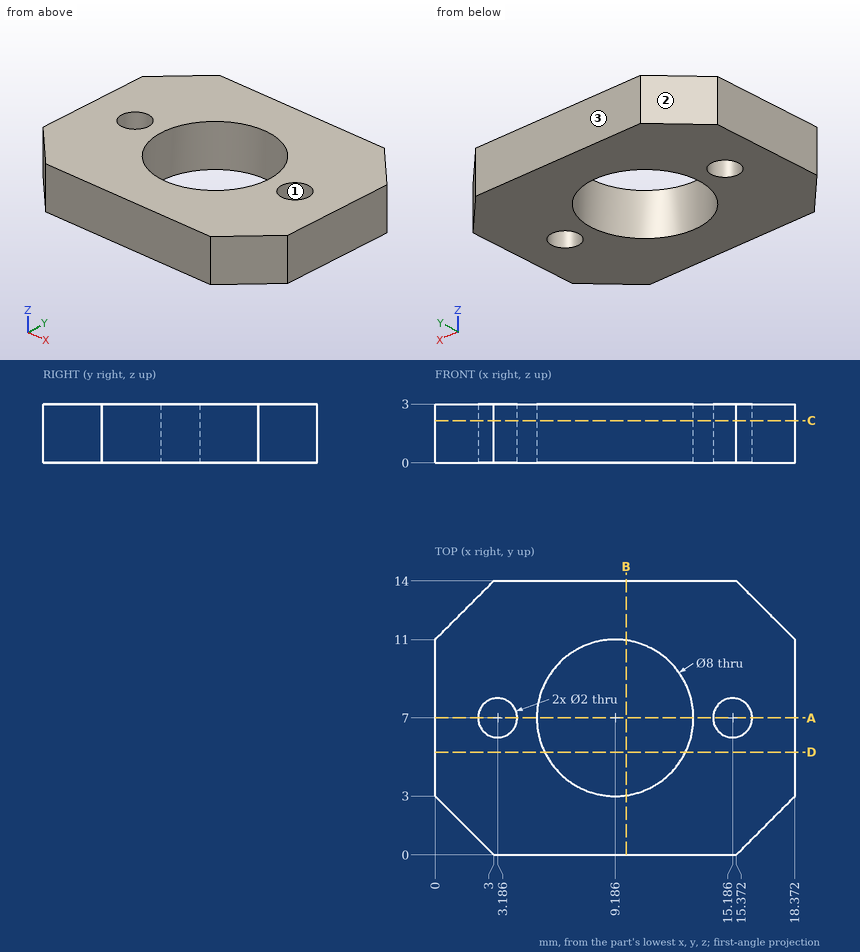
For this review, use the dimensioned drawing (mm, ordinates from the lowest corner) and the shaded views. Give positions to 0.01 mm unless a question says otherwise; leave off trailing zeros. Order: outer loops, then holes, each group sorted by start corner. A loop starts at its lowest first (then second) coordinate and runs counter-clockwise, first axis right, second up. Notation, with made-up numbers: (72.5, 82) - (86.5, 82) arc R19 ccw to (86.5, 110) - close; hole circle Ø10 at (35.25, 17.5). An arc over 180 degrees is marked (long way). Write item = value, one per line. Start each with the question number.
Q1. We need section D-D on y = 5.25. State the section outline as (x, z) points, plus the area to 3 significant figures.
Q2. Clearance check with flat-ended pins moving along their axes: pin 1 Ø2.5 at (x, y) = (15.19, 7) entering from +Z; pin 2 Ø1.6 at (x, y) = (3.19, 7) entering from -Z. State where each tip first meets the part, or that it passes through.
Q3. We need section A-A on y = 7. State the section outline as (x, z) points.
Q4. Mouldability with a two-part tool opening along X and no side actions: class the marked faces 1, 2 and 3 as released by +X, released by -X, zero draft, split by the parting line, or undercut.
Q5. We need section B-B on x = 9.75. State the section outline as (y, z) points, plus the area to 3 significant figures.
Q6. We need section C-C on z = 2.15. State the section outline as (x, y) points.
Q7. To check wall thickness, follow L1, parallel to X at y = 7.25, z = 1.6; L2, parallel to X at y = 9.75, z = 2.3; L3, parallel to Y at x = 8, z = 1.3. State the ranges of each line that lie inside material, in increasing order. Write a range as from..to.
Working result:
q1.outline = (0, 0) - (5.59, 0) - (5.59, 3) - (0, 3) - close; (12.78, 0) - (18.37, 0) - (18.37, 3) - (12.78, 3) - close
q1.area = 33.5 mm²
q2.pin_1 = 3
q2.pin_2 = through
q3.outline = (0, 0) - (2.19, 0) - (2.19, 3) - (0, 3) - close; (4.19, 0) - (5.19, 0) - (5.19, 3) - (4.19, 3) - close; (13.19, 0) - (14.19, 0) - (14.19, 3) - (13.19, 3) - close; (16.19, 0) - (18.37, 0) - (18.37, 3) - (16.19, 3) - close
q4.face_1 = undercut
q4.face_2 = released by -X
q4.face_3 = zero draft
q5.outline = (0, 0) - (3.04, 0) - (3.04, 3) - (0, 3) - close; (10.96, 0) - (14, 0) - (14, 3) - (10.96, 3) - close
q5.area = 18.2 mm²
q6.outline = (0, 3) - (3, 0) - (15.37, 0) - (18.37, 3) - (18.37, 11) - (15.37, 14) - (3, 14) - (0, 11) - close; hole circle Ø2 at (3.19, 7); hole circle Ø8 at (9.19, 7); hole circle Ø2 at (15.19, 7)
q7.L1 = 0..2.22, 4.15..5.19, 13.18..14.22, 16.15..18.37
q7.L2 = 0..6.28, 12.09..18.37
q7.L3 = 0..3.18, 10.82..14
